Could you check a few things on this drawing? It's one solid part, dimensions in mm from its lowest x, y, z. Round coordinates to 2 decimals unless told otherwise and drop trailing zeros. Write each loop counter-clockwise with the first axis right and the second up, starting at its lowest first coordinate (ties: lowest second). Pieces come first, ordered by that corner, then holes. Notation, with made-up numbers: (27.5, 13.5) -> (74.5, 13.5) arc R26 cw to (74.5, 30.5) -> close; hole circle Ø4 at (43.5, 40). An arc over 180 degrees is marked (long way). Answer as CSV lines item,"result".
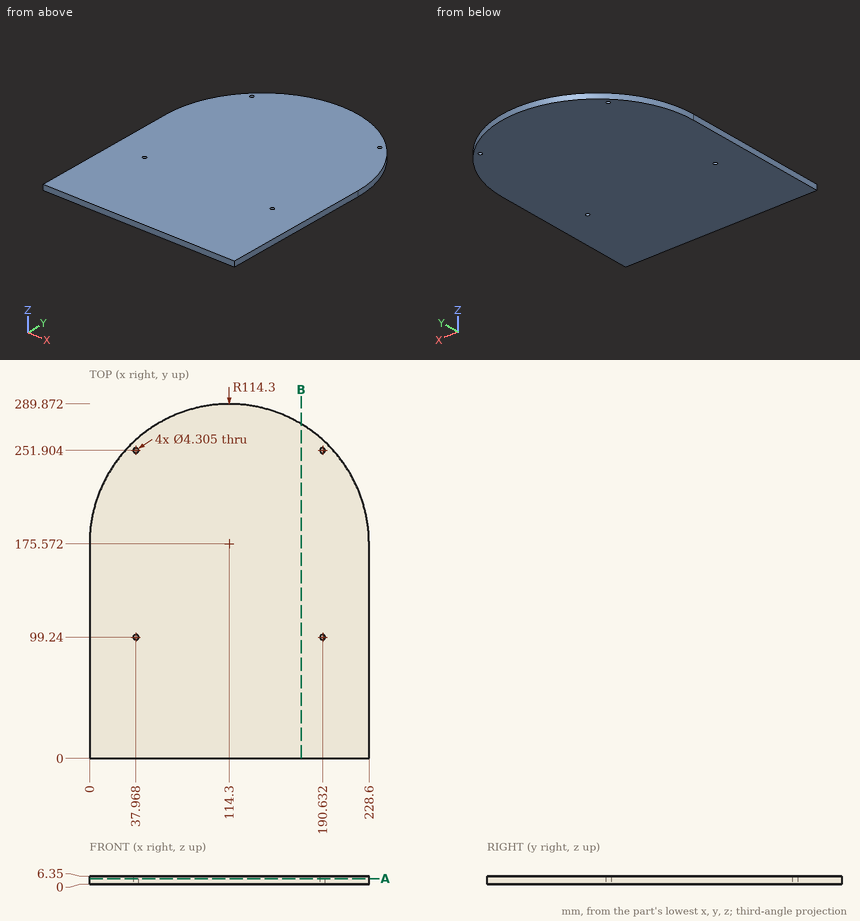
1. For pin 1 Ø1.5 at (x, z) = (151.5, 5.5) entering from +Y, with a flat end and sliding along its axis, tell me the tip position at first contact or that it passes through.
Numbers:
pin 1,"stops at y = 283.9"
2. Suppose I cut it at B-B on x = 173. Please give me the cut outline in (y, z).
Numbers:
outline,"(0, 0) -> (273.65, 0) -> (273.65, 6.35) -> (0, 6.35) -> close"
3. If I drill on line 1 (X direction, y = 98.5, z = 1.25) (1 decimal); line 2 (Y direction, x = 115, z = 1); line 3 (Y direction, x = 117.5, z = 3.5), over which ranges is the centre line in solid material (lowest first)?
Numbers:
line 1,"x = 0 to 35.9, 40 to 188.6, 192.7 to 228.6"
line 2,"y = 0 to 289.87"
line 3,"y = 0 to 289.83"
4. Suppose I cut it at A-A on z = 4.5. Please give me the cut outline in (x, y) (1 decimal), and give its area (3 significant figures).
Numbers:
outline,"(0, 0) -> (228.6, 0) -> (228.6, 175.6) arc R114.3 ccw to (0, 175.6) -> close; hole circle Ø4.3 at (38, 99.2); hole circle Ø4.3 at (38, 251.9); hole circle Ø4.3 at (190.6, 99.2); hole circle Ø4.3 at (190.6, 251.9)"
area,"60,600 mm^2"
